Answer from the drawing. Dimensions are ordinates in mm from the lowest x, y and z of the part. Give positions to 0.01 mm unless a question says otherwise; leave off trailing zeros. Loops run counter-clockwise (first coordinate to the right, second up) from the corner with the lowest first, then second, coordinate; pieces in that order, holes last. Notation, with made-up numbers: (33, 69.25) -> (74, 69.25) arc R19 ccw to (74, 85.25) -> close; hole circle Ø3 at (46.5, 60). An arc over 180 degrees is marked (long way). Write each question's results on one line, items separated by ' | '. Start each with the question number.
Item 1: This flat-tipped pin is pushed along its axis until it touches: P1, Ø6, axis at x = 30, z = 20, coming from the +Y side. Where does it stop, or does it pass through?
Item 2: Section A-A on z = 140 is taken. Write down the section's boundary in (x, y), and give its area (3 significant figures).
Item 3: Section B-B on x = 30 is taken. Write down the section's boundary in (y, z).
Item 4: Find the intervals of material crossed by line 1 (X direction, y = 5.5, z = 140); line 2 (Z direction, x = 210, y = 15.25); line 3 (X direction, y = 5.25, z = 139), in increasing order.
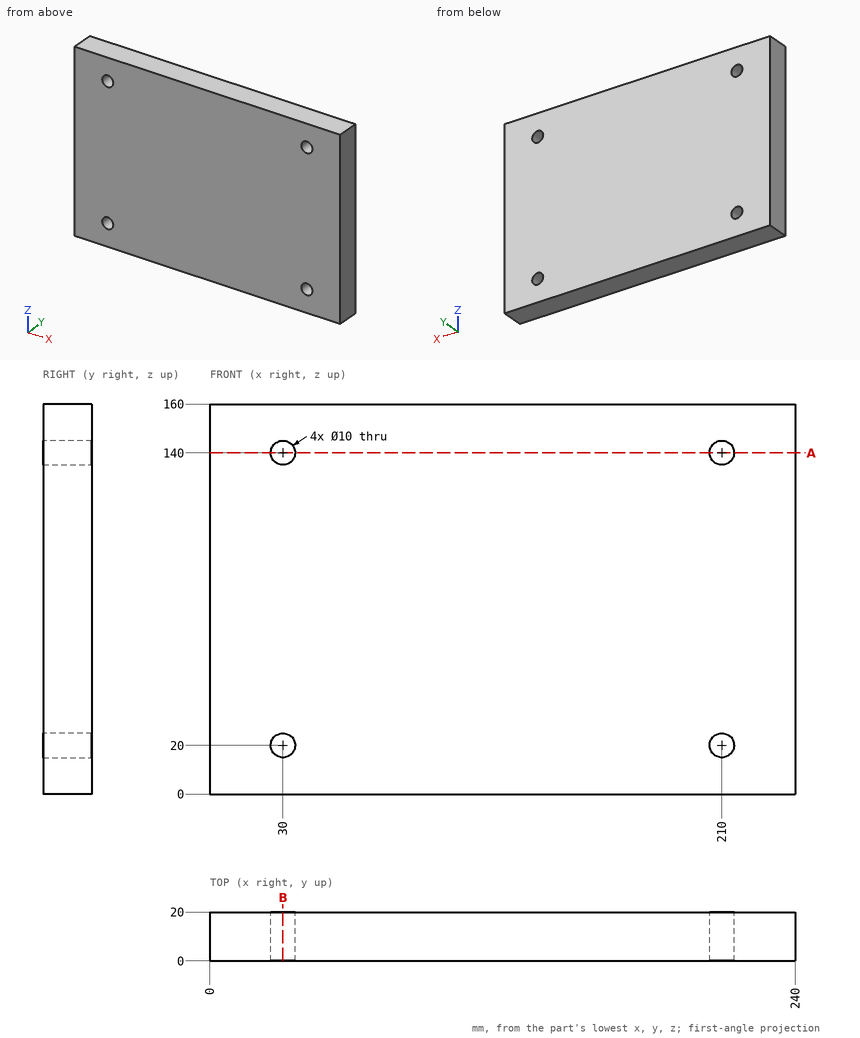
Findings:
1) P1: through
2) outline: (0, 0) -> (25, 0) -> (25, 20) -> (0, 20) -> close; (35, 0) -> (205, 0) -> (205, 20) -> (35, 20) -> close; (215, 0) -> (240, 0) -> (240, 20) -> (215, 20) -> close | area: 4,400 mm2
3) outline: (0, 0) -> (20, 0) -> (20, 15) -> (0, 15) -> close; (0, 25) -> (20, 25) -> (20, 135) -> (0, 135) -> close; (0, 145) -> (20, 145) -> (20, 160) -> (0, 160) -> close
4) line 1: 0 to 25, 35 to 205, 215 to 240 | line 2: 0 to 15, 25 to 135, 145 to 160 | line 3: 0 to 25.1, 34.9 to 205.1, 214.9 to 240
